Autodesk Inventor part; units mm, degrees
ref_plane "Work Plane1" through (0, 0, 0) normal (0, 0, -1) x (-1, 0, 0)
ref_plane "YZ Plane" through (0, 0, 0) normal (1, 0, 0) x (0, 1, 0)
ref_plane "XZ Plane" through (0, 0, 0) normal (0, 1, 0) x (-1, 0, 0)
sketch "Sketch1" plane through (0, 0, 0) normal (0, 0, 1) x (1, 0, 0)
  line L0 (0, 0) -> (0, 37.8188) construction
  line L1 (0, 0) -> (95.7615, 0) construction
  line L2 (0, 0) -> (261.6228, 0)
  line L3 (0, 0) -> (0, 70)
  arc A0 (261.6228, 0) -> (261.6228, 70) centre (261.6228, 35) ccw
  line L4 (261.6228, 70) -> (0, 70)
  dimension "d10" = 35
extrude "Extrusion1" add sketch "Sketch1" along normal mid plane 75
sketch "Sketch2" plane through (0, 0, 37.5) normal (-1, 0, 0) x (0, 0, 1)
  circle A0 centre (-37.5, 35) radius 12.5
  line L0 (0, 70) -> (0, 0)
  line L1 (0, 0) -> (-75, 0)
  point P0 (-37.5, 0)
  point P1 (-37.5, 0)
  dimension "d12" = 25
  dimension "d13" = 35
extrude "Extrusion2" add sketch "Sketch2" along normal blind 10
ref_plane "Work Plane1" through (0, 0, 0) normal (0, 0, -1) x (-1, 0, 0)
sketch "Sketch3" plane through (0, 0, 0) normal (0, 0, -1) x (-1, 0, 0)
  circle A0 centre (-261.6228, 35) radius 35
  arc A1 (-261.6228, 70) -> (-261.6228, 0) centre (-261.6228, 35) ccw
  point P0 (0, 0)
  dimension "d18" = 70
extrude "Extrusion3" cut sketch "Sketch3" along normal mid plane 50
sketch "Sketch4" plane through (0, 0, 37.5) normal (0, 0, 1) x (1, 0, 0)
  line L0 (0, 70) -> (0, 0)
  line L1 (0, 70) -> (100, 70)
  line L2 (100, 70) -> (100, 80)
  line L3 (100, 80) -> (0, 80)
  line L4 (0, 80) -> (0, 70)
  dimension "d21" = 100
  dimension "d22" = 10
extrude "Extrusion4" add sketch "Sketch4" against normal blind 75
sketch "Sketch5" plane through (0, 0, 37.5) normal (0, 0, 1) x (1, 0, 0)
  line L0 (261.6228, 70) -> (100, 70)
  line L1 (100, 70) -> (211.6228, 70)
  line L2 (211.6228, 70) -> (211.6228, 45)
  line L3 (211.6228, 45) -> (100, 45)
  line L4 (100, 45) -> (100, 70)
  point P0 (0, 0)
  dimension "d25" = 25
  dimension "d28" = 50
extrude "Extrusion5" cut sketch "Sketch5" against normal blind 10
sketch "Sketch6" plane through (0, 0, -37.5) normal (0, 0, -1) x (-1, 0, 0)
  line L0 (-100, 70) -> (-261.6228, 70)
  line L1 (-211.6228, 45) -> (-100, 45)
  line L2 (-100, 70) -> (-211.6228, 70)
  line L3 (-211.6228, 70) -> (-211.6228, 45)
  line L4 (-211.6228, 45) -> (-100, 45)
  line L5 (-100, 45) -> (-100, 70)
  point P0 (0, 0)
extrude "Extrusion6" cut sketch "Sketch6" against normal blind 10
sketch "Sketch7" plane through (261.6228, 70, 25) normal (0, 1, 0) x (1, 0, 0)
  line L0 (-161.6228, -12.5) -> (-161.6228, 62.5)
  line L1 (-50, 52.5) -> (-161.6228, 52.5)
  line L2 (-161.6228, -2.5647) -> (-50, -2.5647)
  line L3 (-50, -2.5647) -> (-50, 52.5)
  line L4 (-50, 52.5) -> (-161.6228, 52.5)
  line L5 (-161.6228, 52.5) -> (-161.6228, -2.5647)
  point P0 (-261.6228, 25)
extrude "Extrusion7" cut sketch "Sketch7" against normal blind 5
fillet "Fillet1" radius 25 2 edges at (50, 80, 37.5) (50, 80, -37.5)
properties material "ABS Plastic"
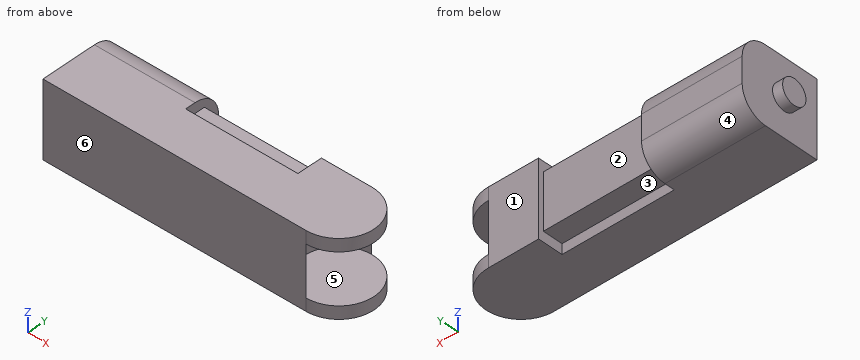
The listing builds one solid part. Answer for the finished solid, in the listing's coordinates (mm). Face numbers are marked on the shaded views. A direction names the side the tool comes from. Give positions to 0.01 mm unless a question says otherwise; leave off trailing zeros. Loops run counter-clockwise (first coordinate to the right, second up) from the corner with the lowest first, then second, coordinate; pieces in that order, holes last.
Item 1: A cutting plane is placed at C-C (x = 177). Give the vertices of the cut face in (y, z), then the cut area to 4 significant figures.
Derived:
outline: (0, -37.5) - (45, -37.5) - (45, -27.5) - (65, -27.5) - (65, 27.5) - (45, 27.5) - (45, 37.5) - (0, 37.5) - close
area: 4,475 mm2
Item 2: A cutting plane is placed at D-D (z = 18). Give the vertices of the cut face in (x, y), then the cut area to 3 significant figures.
Derived:
outline: (0, 0) - (261.62, 0) arc R35 cw to (261.62, 70) - (211.62, 70) - (211.62, 65) - (100, 65) - (100, 79.39) - (0, 79.39) - close
area: 16,800 mm2
Item 3: A cutting plane is placed at B-B (y = 35). Give the vertices of the cut face in (x, z), then the cut area to 3 significant figures.
Derived:
outline: (-10, -12.5) - (0, -12.5) - (0, -37.5) - (296.62, -37.5) - (296.62, -25) - (226.62, -25) - (226.62, 25) - (296.62, 25) - (296.62, 37.5) - (0, 37.5) - (0, 12.5) - (-10, 12.5) - close
area: 19,000 mm2
Item 4: A tool of negligible diameter and unlimited length cuts with its end or side. For the marked faces 1, 2 and 3, from which of +Z, -Z, +X, -X, +Y, -Y can it reach the whole face along a straight path? Write none if from no direction.
Derived:
face 1: +Z, -Z, +X, +Y
face 2: +Z, -Z, +Y
face 3: -Z, +Y
Item 5: Each of these flat-tipped pins is pushed along its axis until it touches: pin 1 Ø5 at (x, z) = (164.5, 31.5) entering from +Y; pin 2 Ø4 at (x, y) = (211.5, 66.5) entering from -Z; pin 3 Ø8 at (x, z) = (241, 22) entering from +Y; pin 4 Ø20 at (y, z) = (63, 0) entering from -X. Where does it stop, or does it pass through?
Derived:
pin 1: stops at y = 45
pin 2: stops at z = -37.5
pin 3: stops at y = 70
pin 4: stops at x = 0
Item 6: A cutting plane is placed at A-A (z = 0). Give the vertices of the cut face in (x, y).
Derived:
outline: (-10, 22.5) - (0, 22.5) - (0, 0) - (261.62, 0) arc R35 cw to (261.62, 70) - (211.62, 70) - (211.62, 65) - (100, 65) - (100, 80) - (0, 80) - (0, 47.5) - (-10, 47.5) - close
Item 7: Find the intervals of material crossed by line 1 along Z through (x, y) = (263, 11); line 2 along X through (y, z) = (73, 15); line 3 along Y through (x, z) = (217, 23.5), in increasing order.
Derived:
line 1: z = -37.5 to -25, 25 to 37.5
line 2: x = 0 to 100
line 3: y = 0 to 70
Item 8: Determine the mould class of the marked faces 4, 5 and 6 for opening direction Z: +Z half, -Z half, draft (parallel to the pull), parting line (faces both ways), or undercut.
Derived:
face 4: -Z half
face 5: undercut
face 6: draft
